Print and shaded views of the part. All mm, measured from the part's lowest x, y and z. A direction names the side the tool comes from. Round coordinates to 2 decimals unless told otherwise and drop trailing zeros. Write each loop counter-clockwise with the first axis right and the second up, starting at its lowest first coordinate (ties: lowest second). Pieces come first, ordered by that corner, then holes. Notation, with made-up numbers: (74, 49.5) - (83, 49.5) arc R12 ccw to (83, 65.5) - close; hole circle Ø8 at (0.25, 15). An arc over 180 degrees is marked (long way). Put each result on its own line as item: value. Start each with the question number.
Item 1: Cut at D-D (x = 9.5). Give the cut face in (y, z) (1 decimal).
Item 2: Drill centre lines: line 1 (Z direction, x = 1.25, y = 5.75); line 2 (Y direction, x = 3.75, z = 37.5) (1 decimal); line 3 (Z direction, x = 5.5, y = 3.75). Where is each one in solid material? Low to high. Write a range as from..to.
Item 3: 3-axis set-ups, long thin cutter, end or side, ignore diameter. For the marked faces 3 and 4: which of +Z, -Z, +X, -X, +Y, -Y reach the whole face in a straight line?
Item 4: Cut at B-B (y = 5.25). Count the separate pieces of the cut face and the enclosed holes in it.
Item 5: Cut at C-C (z = 3.5). Give the cut face in (x, y) (1 decimal).
Item 6: Pin check, flat tips, straight feed: pin 1 Ø1.4 at (x, y) = (4, 6.5) entering from -Z; pin 2 Ø1.8 at (y, z) = (5.715, 13.875) entering from +X; pin 3 Ø2.5 at (x, y) = (4, 6.5) entering from +Z; pin 4 Ø6 at (x, z) = (20, 5) entering from +Y (1 decimal). Stop position of each tip, or through.
Item 7: Mould opens along Z. For the marked faces 1 and 2 say: released by +Z, released by -Z, zero draft, split by the parting line, or undercut.
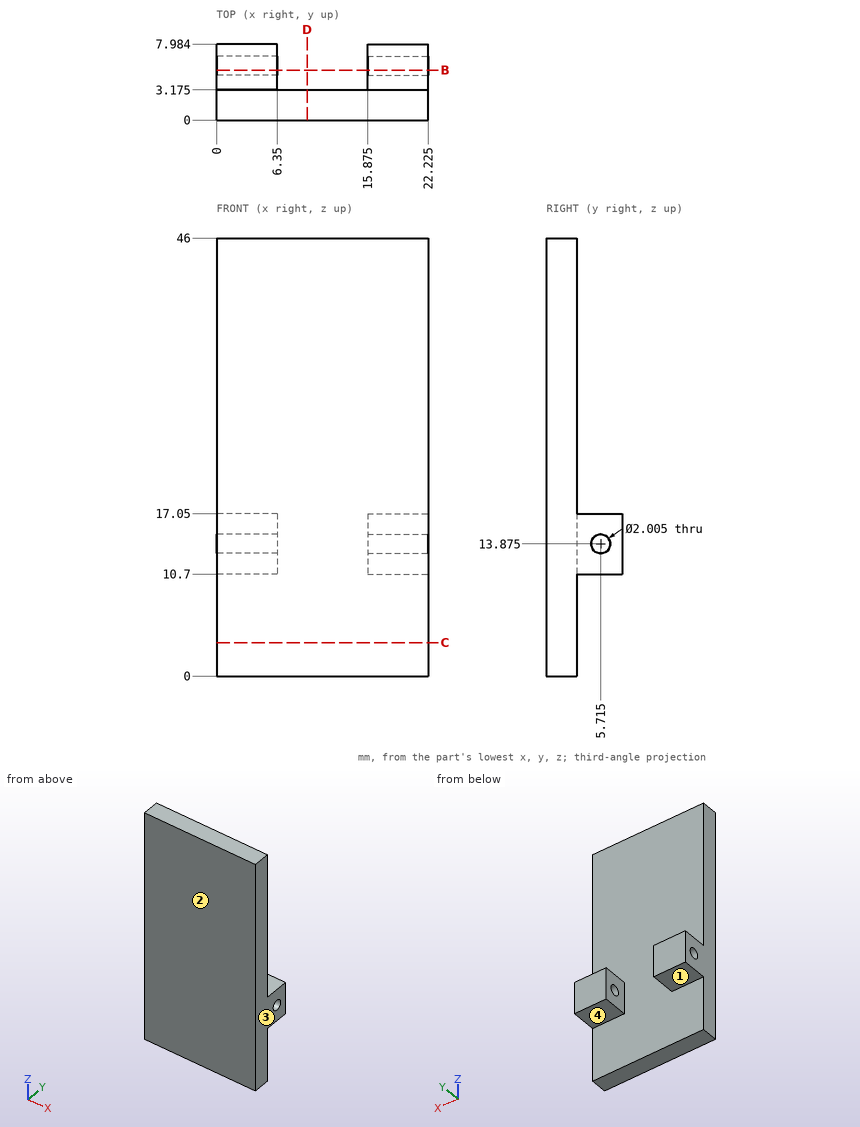
Output values:
1. outline: (0, 0) - (3.2, 0) - (3.2, 46) - (0, 46) - close
2. line 1: 10.7..12.87, 14.88..17.05
2. line 2: 0..3.2
2. line 3: 10.7..17.05
3. face 3: +Z, -Z, +X, +Y, -Y
3. face 4: -Z, +X, -X, +Y
4. separate pieces: 4
4. enclosed holes: 0
5. outline: (0, 0) - (22.2, 0) - (22.2, 3.2) - (0, 3.2) - close
6. pin 1: z = 10.7
6. pin 2: through
6. pin 3: z = 17.05
6. pin 4: y = 3.2
7. face 1: released by -Z
7. face 2: zero draft
